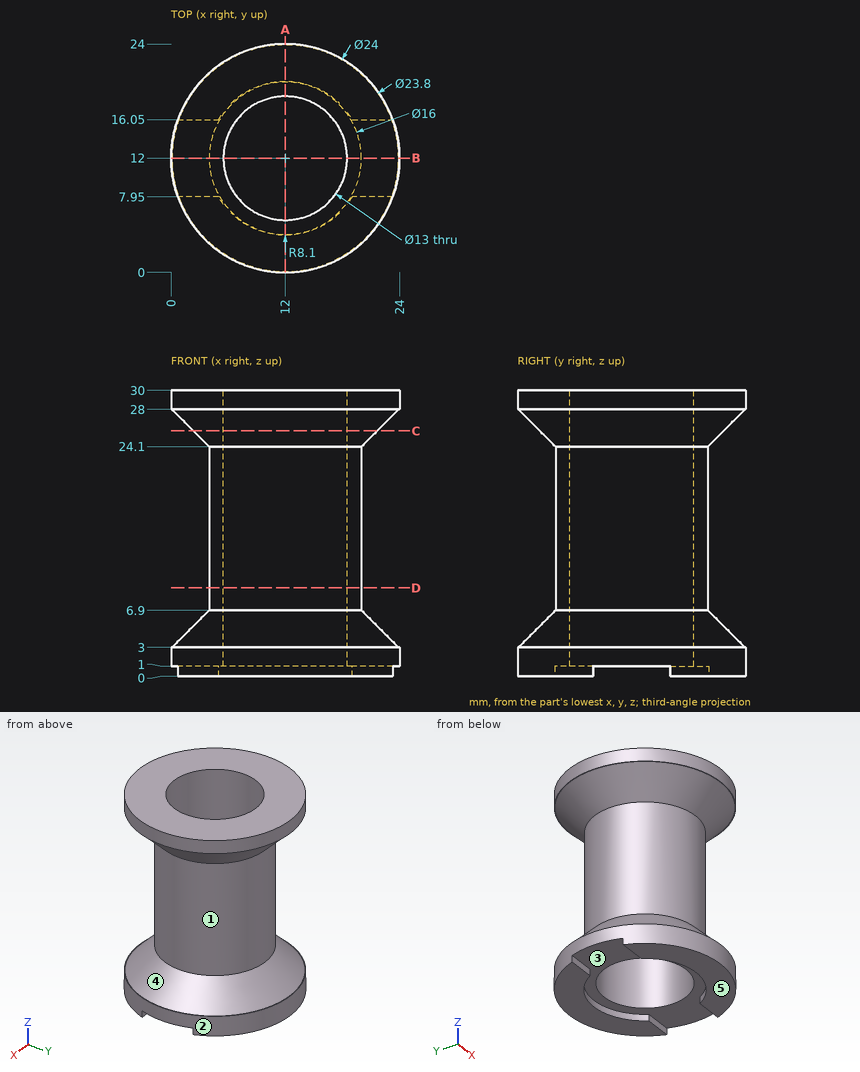
Study the drawing (mm; zero at the part's minimum x, y, z) and answer. A direction names the side the tool comes from. Coordinates: 2 decimals unless noted, no trailing zeros. Loops run counter-clockwise (first coordinate to the right, second up) from the corner with the lowest first, then second, coordinate; pieces in that order, holes last. Notation, with made-up numbers: (43, 70.25) -> (48, 70.25) arc R9 ccw to (48, 87.25) -> close; hole circle Ø9 at (79.5, 26). An arc over 180 degrees is marked (long way). Answer in a Markdown table with one row per item. Add a question column.
1. The part is cut by section D-D, the plane z = 9.25. Write down the section's boundary in (x, y).
2. Determine the mould class of the marked faces 3, 4 and 5 for opening direction X: +X half, -X half, draft (parallel to the pull), parting line (faces both ways), or undercut.
3. The part is cut by section A-A, the plane x = 12. Write down the section's boundary in (y, z).
4. Consider line 1 (Y direction, x = 12, z = 23); line 2 (X direction, y = 9.25, z = 12.75); line 3 (Z direction, x = 9.5, y = 2.5). Determine where each line is inside the solid, lowest interval first. Write a range as [from, to].
5. For the marked faces 1 and 2, determine the directions among +Z, -Z, +X, -X, +Y, -Y from which every point of the face is accessible in a straight line to the end or side of a thin tool.
6. The part is cut by section B-B, the plane y = 12. Write down the section's boundary in (x, z).
7. Flat-ended cylindrical pins translate along their axes: P1, Ø1, axis at x = 18, z = 6.5, coming from the -Y side; P2, Ø2, axis at x = 11, z = 17, coming from the +Y side; P3, Ø8, axis at x = 20, y = 21, coming from the -Z side; P4, Ø0.8, axis at x = 2.5, z = 0.5, coming from the +Y side. Find the tip coordinate at first contact, or state that the pin passes through.
8. The part is cut by section C-C, the plane z = 25.75. Write down the section's boundary in (x, y).
Answer below:
| question | item | result |
|---|---|---|
| 1 | outline | circle Ø16 at (12, 12); hole circle Ø13 at (12, 12) |
| 2 | face 3 | undercut |
| 2 | face 4 | parting line |
| 2 | face 5 | draft |
| 3 | outline | (0, 0) -> (3.9, 0) -> (3.9, 1) -> (5.5, 1) -> (5.5, 30) -> (0, 30) -> (0, 28) -> (0.1, 28) -> (4, 24.1) -> (4, 6.9) -> (0.1, 3) -> (0, 3) -> close; (18.5, 1) -> (20.1, 1) -> (20.1, 0) -> (24, 0) -> (24, 3) -> (23.9, 3) -> (20, 6.9) -> (20, 24.1) -> (23.9, 28) -> (24, 28) -> (24, 30) -> (18.5, 30) -> close |
| 4 | line 1 | [4, 5.5], [18.5, 20] |
| 4 | line 2 | [4.49, 6.11], [17.89, 19.51] |
| 4 | line 3 | [0, 5.08], [25.92, 30] |
| 5 | face 1 | none |
| 5 | face 2 | +Z, -Z |
| 6 | outline | (0, 1) -> (5.5, 1) -> (5.5, 30) -> (0, 30) -> (0, 28) -> (0.1, 28) -> (4, 24.1) -> (4, 6.9) -> (0.1, 3) -> (0, 3) -> close; (18.5, 1) -> (24, 1) -> (24, 3) -> (23.9, 3) -> (20, 6.9) -> (20, 24.1) -> (23.9, 28) -> (24, 28) -> (24, 30) -> (18.5, 30) -> close |
| 7 | P1 | y = 5.29 |
| 7 | P2 | y = 20 |
| 7 | P3 | z = 0 |
| 7 | P4 | y = 19.82 |
| 8 | outline | circle Ø19.3 at (12, 12); hole circle Ø13 at (12, 12) |
